Autodesk Inventor part; units mm, degrees
ref_plane "YZ Plane" through (0, 0, 0) normal (1, 0, 0) x (0, 1, 0)
ref_plane "XZ Plane" through (0, 0, 0) normal (0, 1, 0) x (-1, 0, 0)
ref_plane "XY Plane" through (0, 0, 0) normal (0, 0, 1) x (1, 0, 0)
sketch "スケッチ1" plane through (0, 0, 0) normal (0, 1, 0) x (-1, 0, 0)
  circle A0 centre (0, 0) radius 20
  circle A1 centre (0, 0) radius 40
  dimension "d0" = 40
  dimension "OD" = 80
extrude "押し出し1" add sketch "スケッチ1" along normal blind 3
sketch "スケッチ8" plane through (0, 0, 0) normal (0, -1, 0) x (1, 0, 0)
  circle A0 centre (-0.0001, 0) radius 23.75
  circle A1 centre (-27.2635, 37.05) radius 3.15
  circle A2 centre (-38.2912, 25.4909) radius 3.15
  circle A3 centre (25.4909, 38.2912) radius 5.525
  circle A4 centre (41.2214, 20.4157) radius 5.525
  circle A5 centre (38.2912, -25.4909) radius 4.65
  circle A6 centre (-35.8447, -17.7527) radius 4.65
  circle A7 centre (-2.548, -39.9188) radius 4.65
  arc A8 (-4.7957, -75.1327) -> (4.7957, 75.1327) centre (0, 0) ccw
  arc A9 (4.7957, 75.1327) -> (-4.7957, -75.1327) centre (0, 0) ccw
  circle A10 centre (-16.7482, -62.9346) radius 4.2164
  circle A11 centre (-39.5574, -51.7347) radius 4.2164
  circle A12 centre (-56.3443, -32.6587) radius 4.2164
  circle A13 centre (-64.5532, -8.6107) radius 4.2164
  circle A14 centre (-62.9346, 16.7482) radius 4.2164
  circle A15 centre (-51.7347, 39.5574) radius 4.2164
  circle A16 centre (-32.6587, 56.3443) radius 4.2164
  circle A17 centre (-8.6107, 64.5532) radius 4.2164
  circle A18 centre (16.7482, 62.9346) radius 4.2164
  circle A19 centre (39.5574, 51.7347) radius 4.2164
  circle A20 centre (56.3443, 32.6587) radius 4.2164
  circle A21 centre (64.5532, 8.6107) radius 4.2164
  circle A22 centre (62.9346, -16.7482) radius 4.2164
  circle A23 centre (51.7347, -39.5574) radius 4.2164
  circle A24 centre (32.6587, -56.3443) radius 4.2164
  circle A25 centre (8.6107, -64.5532) radius 4.2164
  circle A26 centre (-29.3091, 1.8708) radius 2.7051
  circle A27 centre (-16.2747, -24.447) radius 2.7051
  circle A28 centre (13.0344, -26.3178) radius 2.7051
  circle A29 centre (29.3091, -1.8708) radius 2.7051
  circle A30 centre (16.2747, 24.447) radius 2.7051
  circle A31 centre (-13.0344, 26.3178) radius 2.7051
  ellipse E0 centre (0.0001, 0) end of major axis (24.6134, -1.5711) minor radius 24.6634 (1.5711, 24.6133) -> (-1.5711, -24.6133) ccw
  ellipse E1 centre (-0.0001, 0) end of major axis (24.6133, -1.5711) minor radius 24.6634 (-1.5711, -24.6133) -> (1.5711, 24.6133) ccw
  line L0 (-16.2747, -24.447) -> (-0.0001, 0) construction
  line L1 (19.7699, -13.161) -> (-19.77, 13.161) construction
  point P0 (13.161, 19.7699)
  point P1 (-13.1611, -19.7699)
  dimension "d88" = 47.5
hole "穴3" at (-19.77, 0, 13.161) at (13.161, 0, 19.7699) at (19.7699, 0, -13.161) at (-13.1611, 0, -19.7699) direction (0, 1, 0) diameter 3.4 depth 3 countersink diameter 6.3 countersink angle 90
sketch "Sketch11" plane through (0, 3, 0) normal (0, 1, 0) x (1, 0, 0)
  circle A0 centre (-2.548, 39.9188) radius 6.6
  circle A1 centre (-35.8447, 17.7527) radius 6.858
  circle A2 centre (-35.8447, 17.7527) radius 10.858
  circle A3 centre (-2.548, 39.9188) radius 10.858
  point P0 (0, 0)
  dimension "d71" = 4
extrude "Extrusion5" cut sketch "Sketch11" against normal through all contours A0 | A1 | A2 | A3
sketch "Sketch13" plane through (0, 3, 0) normal (0, 1, 0) x (1, 0, 0)
  circle A0 centre (-19.9494, 29.967) radius 2.1
  circle A1 centre (35.9269, 2.2932) radius 2.1
  circle A2 centre (-15.9775, -32.2602) radius 2.1
  circle A3 centre (0, 0) radius 36 construction
  arc A4 (-13.1898, 37.7628) -> (8.2815, 39.1333) centre (-2.548, 39.9188) ccw
  arc A5 (-39.2984, 7.4587) -> (-29.7497, 26.7387) centre (-35.8447, 17.7527) ccw
  line L0 (-2.548, 39.9188) -> (-35.8447, 17.7527) construction
  line L1 (-19.1963, 28.8358) -> (0, 0) construction
  line L2 (0, 0) -> (35.9269, 2.2932) construction
  line L3 (0, 0) -> (-15.9775, -32.2602) construction
  dimension "d83" = 72
  dimension "d84" = 4.2
  dimension "d85" = 120
  dimension "d86" = 120
extrude "Extrusion7" cut sketch "Sketch13" against normal through all
fillet "Fillet2" radius 2 4 edges at (-39.2984, 1.5, -7.4587) (-29.7497, 1.5, -26.7387) (8.2815, 1.5, -39.1333) (-13.1898, 1.5, -37.7628)
properties part number "cathode_jig"
The model under review builds one solid part; all positions refer to its coordinate system, in mm. Give positions to 0.01 mm unless a question says otherwise; leave off trailing zeros. Order: outer loops, then holes, each group sorted by start corner. A loop starts at its lowest first (then second) coordinate and runs counter-clockwise, first axis right, second up. Notation, with made-up numbers: M 17.25,-5.5 L 41.25,-5.5 A29 cw 41.25,22.5 Z; hole C 34,3.25 d3. An arc over 180 degrees is marked long. One line per question, with ' | ' between items. Start each with the question number.
1) Consider section D-D, the plane x = -33. Give the boundary of the cut face in (y, z).
2) Consider section C-C, the plane y = 0.8. State how many separate pieces and enclosed holes the cut face has, then the cut area to 3 significant figures.
3) Consider section B-B, the plane z = 7. Give the boundary of the cut face in (x, y) (3 decimals), then the cut area to 3 significant figures.
4) Clearance check with flat-ended pins moving along their axes: P1, Ø8, axis at x = 30, z = -24, coming from the -Y side; P2, Ø3, axis at x = -13.16, z = -19.77, coming from the -Y side. State where each tip first meets the part, or that it passes through.
5) Wall thickness on L1, parallel to X at y = 1, z = -4; L2, parallel to Z at x = 14, y = 2.1; L3, parallel to Z at x = -12.5, y = 0.9: over which ranges is each line inside the solid? List them lowest first. Write a range as from..to.
6) Consider section A-A, the plane x = 0. Give the boundary of the cut face in (y, z), then the cut area to 3 significant figures.
7) Mouldability with a two-part tool opening along Z and no side actions: class faces 1 (the face through (18, 0, 10)), 2 (the face through (23.22, 1.48, 32.57)), 3 (the face through (-18.736, 2.236, 14.51)), 4 (the face through (-16.251, 1.521, 30.178)) as pulls with the +Z half, pulls with the -Z half, needs draft (parallel to the pull), parting line crosses it, or undercut.
Found:
1) outline: M 0,-7.27 L 3,-7.27 L 3,22.61 L 0,22.61 Z
2) separate pieces: 1 | enclosed holes: 8 | area: 3,310 mm²
3) outline: M -39.383,0 L -18.735,0 L -18.735,3 L -39.383,3 Z; M 18.735,0 L 39.383,0 L 39.383,3 L 18.735,3 Z | area: 124 mm²
4) P1: stops at y = 0 | P2: passes through
5) L1: x = -39.8..-19.6, 19.6..34.7, 37.15..39.8 | L2: z = -37.47..-14.28, 14.28..18.29, 21.25..37.47 | L3: z = -35.58..-21.92, -17.62..-15.61, 15.61..38
6) outline: M 0,-29.36 L 3,-29.36 L 3,-20 L 0,-20 Z; M 0,20 L 3,20 L 3,40 L 0,40 Z | area: 88.1 mm²
7) face 1: needs draft | face 2: parting line crosses it | face 3: undercut | face 4: undercut
